For this review, take the finished solid that the model builds, in its own axes (mm). A direction names the side the tool comes from. Round coordinates to 2 decimals unless told otherwise and drop trailing zeros. Write each loop counter-clockwise with the first axis right and the second up, starting at its lowest first coordinate (ties: lowest second). Pieces come first, ordered by that corner, then holes.
Autodesk Inventor part; units mm, degrees
ref_plane "YZ Plane" through (0, 0, 0) normal (1, 0, 0) x (0, 1, 0)
ref_plane "XZ Plane" through (0, 0, 0) normal (0, 1, 0) x (-1, 0, 0)
ref_plane "XY Plane" through (0, 0, 0) normal (0, 0, 1) x (1, 0, 0)
sketch "Boceto1" plane through (0, 0, 0) normal (0, 0, 1) x (1, 0, 0)
  line L0 (0, 0) -> (0, 16)
  line L1 (0, 16) -> (-54, 16)
  line L2 (-54, 16) -> (-54, 10)
  line L3 (-54, 10) -> (-29, 10)
  line L4 (0, 0) -> (-39.6047, 0)
  line L5 (-29, 10) -> (-29, 0)
  line L6 (-54, 13.5) -> (-50.5, 13.5)
  line L7 (-50.5, 13.5) -> (-50.5, 10)
  circle A0 centre (-50.5, 13.5) radius 1.25
  line L8 (-50.5, 13.5) -> (-42.5, 13.5)
  line L9 (-42.5, 13.5) -> (-34.5, 13.5)
  circle A1 centre (-42.5, 13.5) radius 1.25
  circle A2 centre (-34.5, 13.5) radius 1.25
  line L10 (0, 0) -> (0, -16)
  line L11 (0, -16) -> (-54, -16)
  line L12 (-54, -16) -> (-54, -10)
  line L13 (-54, -10) -> (-29, -10)
  line L14 (-29, -10) -> (-29, 0)
  circle A3 centre (-50.5, -13.5) radius 1.25
  circle A4 centre (-42.5, -13.5) radius 1.25
  circle A5 centre (-34.5, -13.5) radius 1.25
  point P0 (-54, -13.5)
  point P1 (-50.5, 12.25)
  point P2 (-51.75, 13.5)
  dimension "d0" = 10
  dimension "d1" = 25
  dimension "d2" = 6
  dimension "d3" = 54
  dimension "d4" = 3.5
  dimension "d5" = 3.5
  dimension "d6" = 2.5
  dimension "d7" = 8
  dimension "d8" = 8
  dimension "d9" = 2.5
  dimension "d10" = 2.5
extrude "Extrusión1" add sketch "Boceto1" along normal blind 6 contours L4 L5 L3 L7 A0 L6 L2 L1 L0 | L10 L11 L12 L13 L14 L4 | L6 A0 L7 L3 L2
sketch "Boceto2" plane through (0, 0, 6) normal (0, 0, 1) x (1, 0, 0)
  circle A0 centre (-50.5, 13.5) radius 1.25
  line L0 (-50.5, 13.5) -> (-20, 13.5)
  line L1 (-54, 10) -> (-29, 10)
  line L2 (-20, 13.5) -> (-20, 0)
  point P0 (0, 0)
  dimension "d13" = 30.5
hole "Agujero1" at (-20, 0, 6) direction (0, 0, -1) diameter 11.5 end through all
properties part number "Sopoter_gripperM"
(1) For pin 1 Ø3 at (y, z) = (6, 3.5) entering from -X, flat-tipped, find the tip position at first contact; note if it passes through.
Geometry check:
pin 1: stops at x = -29
(2) We need section D-D, the plane x = -34.5. Give the boundary of the cut face in (y, z), and give its area (3 significant figures).
Geometry check:
outline: (-16, 0) - (-14.75, 0) - (-14.75, 6) - (-16, 6) - close; (-12.25, 0) - (-10, 0) - (-10, 6) - (-12.25, 6) - close; (10, 0) - (12.25, 0) - (12.25, 6) - (10, 6) - close; (14.75, 0) - (16, 0) - (16, 6) - (14.75, 6) - close
area: 42.0 mm2
(3) Mouldability with a two-part tool opening along Y and no side actions: class faces 3 (the face through (-29, 0, 3)), 4 (the face through (-27, -16, 3)), 5 (the face through (-27, 0, 6)) as pulls with the +Y half, pulls with the -Y half, needs draft (parallel to the pull), parting line crosses it, or undercut.
Geometry check:
face 3: undercut
face 4: pulls with the -Y half
face 5: needs draft
(4) We need section B-B, the plane y = 13.5. Give the boundary of the cut face in (x, z).
Geometry check:
outline: (-54, 0) - (-51.75, 0) - (-51.75, 6) - (-54, 6) - close; (-49.25, 0) - (-43.75, 0) - (-43.75, 6) - (-49.25, 6) - close; (-41.25, 0) - (-35.75, 0) - (-35.75, 6) - (-41.25, 6) - close; (-33.25, 0) - (0, 0) - (0, 6) - (-33.25, 6) - close
(5) For line 1 along X through (y, z) = (13.5, 3.9); line 2 along Y through (x, z) = (-42.5, 2.4); line 3 along Y through (x, z) = (-41, 3.65), list the stretches that pass through material, from the lowest coordinate up.
Geometry check:
line 1: x = -54 to -51.75, -49.25 to -43.75, -41.25 to -35.75, -33.25 to 0
line 2: y = -16 to -14.75, -12.25 to -10, 10 to 12.25, 14.75 to 16
line 3: y = -16 to -10, 10 to 16
(6) We need section A-A, the plane x = -20. Give the boundary of the cut face in (y, z), and give its area (3 significant figures).
Geometry check:
outline: (-16, 0) - (-5.75, 0) - (-5.75, 6) - (-16, 6) - close; (5.75, 0) - (16, 0) - (16, 6) - (5.75, 6) - close
area: 123 mm2
(7) We need section C-C, the plane z = 3.9. Give the boundary of the cut face in (x, y).
Geometry check:
outline: (-54, -16) - (0, -16) - (0, 16) - (-54, 16) - (-54, 10) - (-29, 10) - (-29, -10) - (-54, -10) - close; hole circle Ø2.5 at (-50.5, -13.5); hole circle Ø2.5 at (-50.5, 13.5); hole circle Ø2.5 at (-42.5, -13.5); hole circle Ø2.5 at (-42.5, 13.5); hole circle Ø2.5 at (-34.5, -13.5); hole circle Ø2.5 at (-34.5, 13.5); hole circle Ø11.5 at (-20, 0)
(8) For faces 1 (the face through (-43.75, -13.55, 2.96)), 2 (the face through (-42, -10, 3)), list the 3-axis set-ups (+Z, -Z, +X, -X, +Y, -Y) from which the entire face can be reached by the end or side of a thin tool; tool diameter is ignored.
Geometry check:
face 1: +Z, -Z
face 2: +Z, -Z, -X
